Model file for the job. Use its own axes, mm. Round coordinates to 2 decimals unless told otherwise and drop trailing zeros. Write each loop counter-clockwise with the first axis right and the second up, starting at its lowest first coordinate (ties: lowest second). Pieces come first, ordered by that corner, then holes.
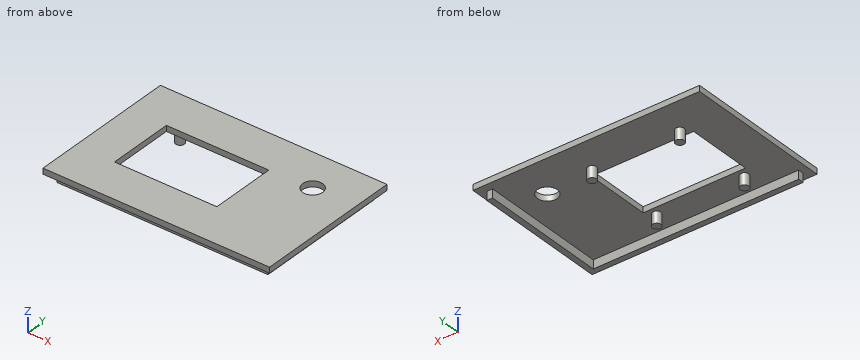
```python
from build123d import *

# Parameters (mm, degrees)
SKIZZE10_W                       = 79
SKIZZE10_H                       = 52
AUFSATZ_LINEAR_AUSTRAGEN8_DEPTH  = 2
SKIZZE11_W                       = 35.7
SKIZZE11_H                       = 23
SCHNITT_LINEAR_AUSTRAGEN3_DEPTH  = 2
SKIZZE13_R                       = 3.5
SCHNITT_LINEAR_AUSTRAGEN4_DEPTH  = 2
SKIZZE14_R                       = 1.5
AUFSATZ_LINEAR_AUSTRAGEN9_DEPTH  = 4
AUFSATZ_LINEAR_AUSTRAGEN10_DEPTH = 3


with BuildPart() as part:
    # Skizze10 → Aufsatz-Linear austragen8 (new body)
    with BuildSketch(Plane.XY):
        with Locations((-19.990421456, -28.402298851)):
            Rectangle(SKIZZE10_W, SKIZZE10_H)
    extrude(amount=AUFSATZ_LINEAR_AUSTRAGEN8_DEPTH)

    # Skizze11 → Schnitt-Linear austragen3 (cut)
    with BuildSketch(Plane.XY.offset(2)):
        with Locations((-28.136972684, -28.402298851)):
            Rectangle(SKIZZE11_W, SKIZZE11_H)
    extrude(amount=-SCHNITT_LINEAR_AUSTRAGEN3_DEPTH, mode=Mode.SUBTRACT)

    # Skizze13 → Schnitt-Linear austragen4 (cut)
    with BuildSketch(Plane.XY.offset(2)):
        with Locations((4.61130293, -16.402298851)):
            Circle(SKIZZE13_R)
    extrude(amount=-SCHNITT_LINEAR_AUSTRAGEN4_DEPTH, mode=Mode.SUBTRACT)

    # Skizze14 → Aufsatz-Linear austragen9 (add)
    with BuildSketch(Plane(origin=(0, 0, 0), x_dir=(-1, 0, 0), z_dir=(0, 0, -1))):
        with Locations((43.436972684, -14.102298851)):
            Circle(SKIZZE14_R)
        with Locations((43.436972684, -42.702298851)):
            Circle(SKIZZE14_R)
        with Locations((12.836972684, -14.102298851)):
            Circle(SKIZZE14_R)
        with Locations((12.836972684, -42.702298851)):
            Circle(SKIZZE14_R)
    extrude(amount=AUFSATZ_LINEAR_AUSTRAGEN9_DEPTH)

    # Skizze15 → Aufsatz-Linear austragen10 (add)
    with BuildSketch(Plane(origin=(0, 0, 0), x_dir=(-1, 0, 0), z_dir=(0, 0, -1))):
        Polygon((-16.809578544, -5.102298851), (-16.809578544, -51.702298851), (56.790421456, -51.702298851), (56.790421456, -49.702298851), (-14.809578544, -49.702298851), (-14.809578544, -5.102298851), align=None)
    extrude(amount=AUFSATZ_LINEAR_AUSTRAGEN10_DEPTH)


solid = part.part
```
1) Cut at C-C on z = -1.65. List the corners of the cut face in (x, y), and give its area (3 significant figures).
2) Cut at A-A on x = -27.5. List the corners of the cut face in (y, z), and give its area (3 significant figures).
3) Cut at B-B on y = -37. List the corners of the cut face in (x, z).
4) Flat gauge pins, fed straight in: pin 1 Ø6.5 at (x, y) = (4.61, -16.4) entering from +Z; pin 2 Ø15.5 at (x, y) = (-11, -26) entering from -Z; pin 3 Ø1 at (x, z) = (-19.5, -1.5) entering from -Y; pin 4 Ø3 at (x, z) = (-6, -3.5) entering from +Y. Where does each tip first touch, or does it go through?
5) Cut at D-D on y = -46. List the corners of the cut face in (x, z), and give its area (3 significant figures).
6) Wall check: probe 1 along Y at (x, z) = (-25, 1.6); probe 2 along X at (y, z) = (-29, 0.7); probe 3 along Y at (x, z) = (15, -1.35). Give the ranges that are in metal, low to high.
Result sheet:
1. outline: (-56.79, -51.7) - (16.81, -51.7) - (16.81, -5.1) - (14.81, -5.1) - (14.81, -49.7) - (-56.79, -49.7) - close; circle Ø3 at (-43.44, -42.7); circle Ø3 at (-43.44, -14.1); circle Ø3 at (-12.84, -42.7); circle Ø3 at (-12.84, -14.1)
1. area: 265 mm2
2. outline: (-54.4, 0) - (-51.7, 0) - (-51.7, -3) - (-49.7, -3) - (-49.7, 0) - (-39.9, 0) - (-39.9, 2) - (-54.4, 2) - close; (-16.9, 0) - (-2.4, 0) - (-2.4, 2) - (-16.9, 2) - close
2. area: 64.0 mm2
3. outline: (-59.49, 0) - (-45.99, 0) - (-45.99, 2) - (-59.49, 2) - close; (-10.29, 0) - (14.81, 0) - (14.81, -3) - (16.81, -3) - (16.81, 0) - (19.51, 0) - (19.51, 2) - (-10.29, 2) - close
4. pin 1: passes through
4. pin 2: stops at z = 0
4. pin 3: stops at y = -51.7
4. pin 4: stops at y = -49.7
5. outline: (-59.49, 0) - (14.81, 0) - (14.81, -3) - (16.81, -3) - (16.81, 0) - (19.51, 0) - (19.51, 2) - (-59.49, 2) - close
5. area: 164 mm2
6. probe 1: y = -54.4 to -39.9, -16.9 to -2.4
6. probe 2: x = -59.49 to -45.99, -10.29 to 19.51
6. probe 3: y = -51.7 to -5.1
